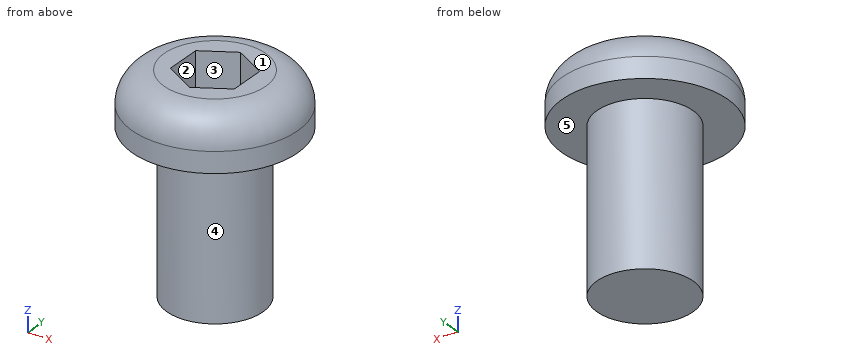
from build123d import *

# Parameters (mm, degrees)
F0_R     = 3
F1_DEPTH = 10
F2_R     = 5.175
F2_R_2   = 3
F3_DEPTH = 3.3
F4_R     = 2
F6_DEPTH = 3


with BuildPart() as f1:
    # F0 (on Top) → F1 (new body)
    with BuildSketch(Plane.XY):
        Circle(F0_R)
    extrude(amount=F1_DEPTH)

    # F2 (on face) → F3 (join)
    with BuildSketch(Plane.XY.offset(10)):
        Circle(F2_R)
        Circle(F2_R_2, mode=Mode.SUBTRACT)
        Circle(F2_R_2)
    extrude(amount=F3_DEPTH)

    # F4
    f4_edges = [f1.edges().sort_by_distance(p)[0] for p in [
        (-5.175, 0, 13.3),
    ]]
    fillet(f4_edges, radius=F4_R)

    # F5 (on face) → F6 (cut)
    with BuildSketch(Plane.XY.offset(13.3)):
        Polygon((2, -1.1547005384), (2, 1.1547005384), (0, 2.3094010768), (-2, 1.1547005384), (-2, -1.1547005384), (0, -2.3094010768), align=None)
    extrude(amount=-F6_DEPTH, mode=Mode.SUBTRACT)


solid = f1.part
The listing builds one solid part. Answer for the finished solid, in the listing's coordinates (mm). Face numbers are marked on the shaded views. A direction names the side the tool comes from. Round coordinates to 2 decimals unless told otherwise and drop trailing zeros. Order: outer loops, then holes, each group sorted by start corner. A loop starts at its lowest first (then second) coordinate and runs counter-clockwise, first axis right, second up. Notation, with made-up numbers: (78, 71) -> (126, 71) arc R28 cw to (126, 104) -> close; hole circle Ø6 at (-36.5, 74.25). An arc over 180 degrees is marked (long way). One line per item, written item: value.
Item 1: For the marked faces 1 and 2, determine the directions among +Z, -Z, +X, -X, +Y, -Y from which every point of the face is accessible in a straight line to the end or side of a thin tool.
Taken from the geometry:
face 1: +Z, +X, -X, +Y, -Y
face 2: +Z
Item 2: Find section B-B, the plane z = 5.25. Give the vertices of the cut face in (x, y), then the cut area to 3 significant figures.
Taken from the geometry:
outline: circle Ø6 at (0, 0)
area: 28.3 mm2
Item 3: Straight lines are drawn through the part: L1, parallel to Z at x = 0.25, y = 2; L2, parallel to X at y = 0.5, z = 11.75; L3, parallel to X at y = -1.5, z = 2. For each, find the intervals that lie inside material, in ascending order.
Taken from the geometry:
L1: z = 0 to 10.3
L2: x = -5.1 to -2, 2 to 5.1
L3: x = -2.6 to 2.6
Item 4: Find section A-A, the plane z = 12. Give the vertices of the cut face in (x, y), then the cut area to 3 significant figures.
Taken from the geometry:
outline: circle Ø10.1 at (0, 0); hole (-2, -1.15) -> (0, -2.31) -> (2, -1.15) -> (2, 1.15) -> (0, 2.31) -> (-2, 1.15) -> close
area: 66.2 mm2
Item 5: For a pull along Y with two mould halves and no side action, classify the marked faces 3, 4 and 5 as released by +Y, released by -Y, zero draft, split by the parting line, or undercut.
Taken from the geometry:
face 3: undercut
face 4: split by the parting line
face 5: zero draft
Item 6: Given P1, Ø1.5, axis at x = 2, z = 2, coming from the -Y side; P2, Ø1.5, axis at y = -0.5, z = 4, coming from the -X side; P3, Ø1.2, axis at y = 0, z = 12.5, coming from the -X side, each flat-ended and moving along its own axis, determine where each tip first touches the part or whether it passes through.
Taken from the geometry:
P1: stops at y = -2.73
P2: stops at x = -3
P3: stops at x = -5.08
